```python
from build123d import *

# Parameters (mm, degrees)
BOSS_EXTRU_1_DEPTH      = 8
ESQUISSE2_R             = 0.625
ENL_V_MAT_EXTRU_2_DEPTH = 8
ENL_V_MAT_EXTRU_4_DEPTH = 8
ESQUISSE4_W             = 2
ESQUISSE4_H             = 7
ENL_V_MAT_EXTRU_6_DEPTH = 8
CONG_4_R                = 1.5
CONG_7_R                = 1.5


with BuildPart() as part:
    # Esquisse1 → Boss.-Extru.1 (new body)
    with BuildSketch(Plane.XY):
        Polygon((-4.284999929, 10.5), (-4.284999929, 3.5), (2.8564285, -3.5), (2.8564285, -10.5), (3.8564285, -10.5), (3.8564285, -3.5), (-3.284999929, 3.5), (-3.284999929, 10.5), align=None)
    extrude(amount=BOSS_EXTRU_1_DEPTH)

    # Esquisse2 → Enlèv. mat.-Extru.2 (cut)
    with BuildSketch(Plane(origin=(-3.284999929, 0, 0), x_dir=(0, 0, -1), z_dir=(1, 0, 0))):
        with Locations(Location((-6, 8.744627622, 0), (0, 0, 90))):
            Circle(ESQUISSE2_R)
        with Locations(Location((-2, 8.744627622, 0), (0, 0, 90))):
            Circle(ESQUISSE2_R)
    extrude(amount=-ENL_V_MAT_EXTRU_2_DEPTH, mode=Mode.SUBTRACT)

    # Esquisse3 → Enlèv. mat.-Extru.4 (cut)
    with BuildSketch(Plane(origin=(0.14, 0.142828569, 0), x_dir=(0.7141428428542851, -0.7, 0), z_dir=(0.7, 0.7141428428542851, 0))):
        Polygon((-4.795959188, -8), (5.204040812, -6), (5.204040812, -8), align=None)
        Polygon((-4.795959188, 0), (5.204040812, -2), (5.204040812, 0), align=None)
    extrude(amount=-ENL_V_MAT_EXTRU_4_DEPTH, mode=Mode.SUBTRACT)

    # Esquisse4 → Enlèv. mat.-Extru.6 (cut)
    with BuildSketch(Plane(origin=(3.8564285, 0, 0), x_dir=(0, 0, -1), z_dir=(1, 0, 0))):
        with Locations((-7, -7)):
            Rectangle(ESQUISSE4_W, ESQUISSE4_H)
        with Locations((-1, -7)):
            Rectangle(ESQUISSE4_W, ESQUISSE4_H)
    extrude(amount=-ENL_V_MAT_EXTRU_6_DEPTH, mode=Mode.SUBTRACT)

    # Congé4
    cong_4_edges = [part.edges().sort_by_distance(p)[0] for p in [
        (3.3564285, -10.5, 2),
    ]]
    fillet(cong_4_edges, radius=CONG_4_R)

    # Congé7
    cong_7_edges = [part.edges().sort_by_distance(p)[0] for p in [
        (3.3564285, -10.5, 6),
    ]]
    fillet(cong_7_edges, radius=CONG_7_R)


solid = part.part
```
Check sheet for the modelled part. Datum: model origin and axes. Units: mm. A direction names the side the tool comes from. Give positions to 0.01 mm unless a question says otherwise; leave off trailing zeros. Order: outer loops, then holes, each group sorted by start corner. A loop starts at its lowest first (then second) coordinate and runs counter-clockwise, first axis right, second up. Notation, with made-up numbers: (76.25, 24.5) -> (87.25, 24.5) arc R28 ccw to (87.25, 46.5) -> close; hole circle Ø9 at (22.5, 86.5). An arc over 180 degrees is marked (long way). Return JSON: item names as keys, results as strings.
1. Set-up check for faces 4 (the flat face through (3.4, -6.3, 6)), 5 (the flat face through (2.856, -7, 4)), 6 (the flat face through (3.4, -6.3, 2)), 7 (the flat face through (-0.006, -0.197, 0.986)), 8 (the flat face through (-3.285, 7, 4)): record each of +Z, -Z, +X, -X, +Y, -Y from which the full face is reachable in a straight line by a thin tool's end or side.
From the geometry:
{"face 4": "+Z, +X, -X, -Y", "face 5": "+Z, -Z, -X, -Y", "face 6": "-Z, +X, -X, -Y", "face 7": "-Z, +X, -Y", "face 8": "+Z, -Z, +X, +Y"}
2. Mould release check, pull along Z, two halves, no side actions. Record for faces 1 (the flat face through (-4, 7, 8)), 2 (the flat face through (-0.46, 0.73, 3.94)), 3 (the cylindrical face through (-3.78, 9.32, 1.76)): +Z half, -Z half, draft (parallel to the pull), parting line (faces both ways), or undercut.
From the geometry:
{"face 1": "+Z half", "face 2": "draft", "face 3": "undercut"}
3. Go/stop test with flat-tipped pins: P1, Ø1.1, axis at y = 8.74, z = 2, coming from the +X side; P2, Ø2, axis at y = 7.5, z = 2.5, coming from the +X side (3 decimals); P3, Ø0.5, axis at x = 3, y = -7.5, coming from the +Z side; P4, Ø2, axis at y = -7, z = 5, coming from the -X side. Record where each tip stops, or that it passes through.
From the geometry:
{"P1": "through", "P2": "x = -3.285", "P3": "z = 6", "P4": "x = 2.86"}
4. Cross-section at B-B, the plane x = -1.75. Record the cut outline in (y, z).
From the geometry:
{"outline": "(1.02, 0.57) -> (2, 0.43) -> (2, 7.57) -> (1.02, 7.43) -> close"}
5. Material ranges on probe 1 along X at (y, z) = (4.5, 3) (3 decimals); probe 2 along Z at (x, y) = (3.25, -7.25); probe 3 along X at (y, z) = (-4, 2.5), recorded low to high. Write a range as [from, to].
From the geometry:
{"probe 1": "[-4.285, -3.285]", "probe 2": "[2, 6]", "probe 3": "[2.86, 3.86]"}
6. Cross-section at A-A, the plane y = 5.75. Record the cut outline in (x, z) (3 decimals), plus the area to 3 significant figures.
From the geometry:
{"outline": "(-4.285, 0) -> (-3.285, 0) -> (-3.285, 8) -> (-4.285, 8) -> close", "area": "8.00 mm^2"}
